from build123d import *

# Parameters (mm, degrees)
SKETCH1_W           = 98
SKETCH1_H           = 96
SKETCH1_W_2         = 73
SKETCH1_H_2         = 1
BOSS_EXTRUDE1_DEPTH = 1
SKETCH2_W           = 73
SKETCH2_H           = 1
BOSS_EXTRUDE2_DEPTH = 5
SKETCH3_W           = 98
SKETCH3_H           = 1
BOSS_EXTRUDE3_DEPTH = 5
SKETCH4_W           = 1
SKETCH4_H           = 10
BOSS_EXTRUDE4_DEPTH = 5
FILLET1_R           = 5
FILLET2_R           = 5
SKETCH5_W           = 1
SKETCH5_H           = 1
CUT_EXTRUDE1_DEPTH  = 5


with BuildPart() as part:
    # Sketch1 → Boss-Extrude1 (new body)
    with BuildSketch(Plane(origin=(0, 0, 0), x_dir=(1, 0, 0), z_dir=(0, 1, 0))):
        with Locations((49, 48)):
            Rectangle(SKETCH1_W, SKETCH1_H)
        with Locations((49, 96.5)):
            Rectangle(SKETCH1_W_2, SKETCH1_H_2)
        with Locations((49, -0.5)):
            Rectangle(SKETCH1_W_2, SKETCH1_H_2)
    extrude(amount=BOSS_EXTRUDE1_DEPTH)

    # Sketch2 → Boss-Extrude2 (add)
    with BuildSketch(Plane(origin=(0, 1, 0), x_dir=(1, 0, 0), z_dir=(0, 1, 0))):
        with Locations((49, -0.5)):
            Rectangle(SKETCH2_W, SKETCH2_H)
        with Locations((49, 96.5)):
            Rectangle(SKETCH2_W, SKETCH2_H)
    extrude(amount=BOSS_EXTRUDE2_DEPTH)

    # Sketch3 → Boss-Extrude3 (add)
    with BuildSketch(Plane(origin=(0, 1, 0), x_dir=(1, 0, 0), z_dir=(0, 1, 0))):
        with Locations((49, 95.5)):
            Rectangle(SKETCH3_W, SKETCH3_H)
        with Locations((49, 0.5)):
            Rectangle(SKETCH3_W, SKETCH3_H)
    extrude(amount=BOSS_EXTRUDE3_DEPTH)

    # Sketch4 → Boss-Extrude4 (add)
    with BuildSketch(Plane(origin=(0, 1, 0), x_dir=(1, 0, 0), z_dir=(0, 1, 0))):
        with Locations((0.5, 71.5)):
            Rectangle(SKETCH4_W, SKETCH4_H)
        with Locations((0.5, 24.5)):
            Rectangle(SKETCH4_W, SKETCH4_H)
        with Locations((97.5, 71.5)):
            Rectangle(SKETCH4_W, SKETCH4_H)
        with Locations((97.5, 24.5)):
            Rectangle(SKETCH4_W, SKETCH4_H)
    extrude(amount=BOSS_EXTRUDE4_DEPTH)

    # Fillet1
    fillet1_edges = [part.edges().sort_by_distance(p)[0] for p in [
        (97.5, 6, -19.5),
        (97.5, 6, -29.5),
    ]]
    fillet(fillet1_edges, radius=FILLET1_R - 0.0001)  # a hair under: the kernel refuses the full size

    # Fillet2
    fillet2_edges = [part.edges().sort_by_distance(p)[0] for p in [
        (0.5, 6, -29.5),
        (0.5, 6, -19.5),
        (0.5, 6, -66.5),
        (0.5, 6, -76.5),
        (97.5, 6, -66.5),
        (97.5, 6, -76.5),
    ]]
    fillet(fillet2_edges, radius=FILLET2_R - 0.0001)  # a hair under: the kernel refuses the full size

    # Sketch5 → Cut-Extrude1 (cut)
    with BuildSketch(Plane(origin=(0, 6, 0), x_dir=(1, 0, 0), z_dir=(0, 1, 0))):
        with Locations((0.5, 0.5)):
            Rectangle(SKETCH5_W, SKETCH5_H)
        with Locations((97.5, 0.5)):
            Rectangle(SKETCH5_W, SKETCH5_H)
        with Locations((97.5, 95.5)):
            Rectangle(SKETCH5_W, SKETCH5_H)
        with Locations((0.5, 95.5)):
            Rectangle(SKETCH5_W, SKETCH5_H)
    extrude(amount=-CUT_EXTRUDE1_DEPTH, mode=Mode.SUBTRACT)


solid = part.part
For this review, take the finished solid that the model builds, in its own axes (mm). A direction names the side the tool comes from. Round coordinates to 2 decimals unless told otherwise and drop trailing zeros. Order: outer loops, then holes, each group sorted by start corner. A loop starts at its lowest first (then second) coordinate and runs counter-clockwise, first axis right, second up. Notation, with made-up numbers: (41, 2) -> (74, 2) arc R9 cw to (74, 11) -> close; hole circle Ø9 at (89, 74). An arc over 180 degrees is marked (long way). Put each result on its own line as item: value.
Q1. Add section C-C on z = -21.5. Write out the cut boundary in (x, y).
Check result:
outline: (0, 0) -> (98, 0) -> (98, 5) -> (97, 5) -> (97, 1) -> (1, 1) -> (1, 5) -> (0, 5) -> close
Q2. Machinability: for faces 1 (the flat face through (92, 3, 0)), 2 (the cylindrical face through (97.51, 4.5, -28.07)), 3 (the flat face through (97, 3, -71)), 4 (the flat face through (6, 3, 0)), 5 (the flat face through (92, 3, -96)), which of the approach directions +Z, -Z, +X, -X, +Y, -Y give a long, thin tool a straight path to every point of the face, cutting with its end or side? Answer none if there is none.
Check result:
face 1: +Z, +X, +Y, -Y
face 2: +X, -X, +Y
face 3: +Y
face 4: +Z, -X, +Y, -Y
face 5: -Z, +X, +Y, -Y
Q3. Add section A-A on x = 40. Write out the cut boundary in (y, z).
Check result:
outline: (0, -97) -> (6, -97) -> (6, -95) -> (1, -95) -> (1, -1) -> (6, -1) -> (6, 1) -> (0, 1) -> close
Q4. Add section B-B on y = 2.5. State how many separate pieces and enclosed holes the cut face has, plus the area to 3 significant figures.
Check result:
separate pieces: 6
enclosed holes: 0
area: 376 mm2
Q5. Insertion check: pin 1 Ø0.5 at (y, z) = (3.5, 0.5) entering from -X; pin 2 Ø3 at (x, y) = (92, 1.5) entering from -Z; pin 3 Ø0.8 at (y, z) = (2.5, -95.5) entering from -X; pin 4 Ø5 at (x, z) = (48, -21) entering from -Y. Each pin has a flat end and moves straight along its axis. Give the tip position at first contact, or say it passes through.
Check result:
pin 1: x = 12.5
pin 2: z = -96
pin 3: x = 1
pin 4: y = 0
Q6. For probe 1 along Z at (x, y) = (9.5, 1.25); probe 2 along Z at (x, y) = (15, 1.5); probe 3 along X at (y, z) = (3.5, -69), list the stretches that pass through material, from the lowest coordinate up. Write a range as [from, to].
Check result:
probe 1: [-96, -95], [-1, 0]
probe 2: [-97, -95], [-1, 1]
probe 3: [0, 1], [97, 98]
Q7. Mouldability with a two-part tool opening along X and no side actions: class faces 6 (the flat face through (97, 3, -24)), 7 (the cylindrical face through (0.51, 4.5, -67.93)), 8 (the flat face through (98, 0.3, -47.3)) as pulls with the +X half, pulls with the -X half, needs draft (parallel to the pull), parting line crosses it, or undercut.
Check result:
face 6: undercut
face 7: needs draft
face 8: pulls with the +X half
Q8. Add section D-D on z = -62.5. Write out the cut boundary in (x, y).
Check result:
outline: (0, 0) -> (98, 0) -> (98, 1) -> (0, 1) -> close
